Part model, mm, in its own coordinate system. Coordinates: 2 decimals unless noted, no trailing zeros. Write each loop counter-clockwise with the first axis right and the second up, starting at its lowest first coordinate (ties: lowest second). Pieces come first, ordered by that corner, then holes. Notation, with made-up numbers: (-27, 16) - (23, 16) arc R22 cw to (23, 47) - close; hole circle Ø10 at (31, 64.5). An arc over 180 degrees is marked (long way). Use one line per item in the form item = value. Start each with the question number.
from build123d import *

# Parameters (mm, degrees)
SKETCH_2_W      = 600
SKETCH_2_H      = 600
EXTRUDE_1_DEPTH = 10
SKETCH_3_R      = 2.5
EXTRUDE_2_DEPTH = 5
SKETCH_4_R      = 5
EXTRUDE_3_DEPTH = 3


with BuildPart() as part:
    # 草图2 → 凸台-拉伸1 (new body)
    with BuildSketch(Plane(origin=(0, 0, 0), x_dir=(1, 0, 0), z_dir=(0, 1, 0))):
        Rectangle(SKETCH_2_W, SKETCH_2_H)
    extrude(amount=EXTRUDE_1_DEPTH)

    # 草图3 → 凸台-拉伸2 (add)
    with BuildSketch(Plane(origin=(0, 10, 0), x_dir=(1, 0, 0), z_dir=(0, 1, 0))):
        with Locations((0, 240)):
            Circle(SKETCH_3_R)
        with Locations((-207.846096908, -120)):
            Circle(SKETCH_3_R)
        with Locations((207.846096908, -120)):
            Circle(SKETCH_3_R)
    extrude(amount=EXTRUDE_2_DEPTH)

    # 草图4 → 凸台-拉伸3 (add)
    with BuildSketch(Plane(origin=(0, 10, 0), x_dir=(1, 0, 0), z_dir=(0, 1, 0))):
        Circle(SKETCH_4_R)
    extrude(amount=EXTRUDE_3_DEPTH)


solid = part.part
Q1. Pin check, flat tip, straight feed: P1, Ø11, axis at x = 1.5, z = -1, coming from the +Y side. Stop position of the tip, or through.
Q2. Slice it at A-A (z = -66.5). List the corners of the cut face in (x, y).
Q3. Drill centre lines: probe 1 along X at (y, z) = (10.5, 120); probe 2 along Y at (x, z) = (185.5, -71.5). Where is each one in solid material? Low to high.
Q4. Slice it at B-B (x = -169). List the corners of the cut face in (y, z), plus the area to 3 significant figures.
Solution:
q1.P1 = 13
q2.outline = (-300, 0) - (300, 0) - (300, 10) - (-300, 10) - close
q3.probe_1 = -210.35 to -205.35, 205.35 to 210.35
q3.probe_2 = 0 to 10
q4.outline = (0, -300) - (10, -300) - (10, 300) - (0, 300) - close
q4.area = 6,000 mm2
